Geometry check sheet. Reference: the model listing, model coordinates, mm. A direction names the side the tool comes from. Round coordinates to 2 decimals unless told otherwise and drop trailing zeros. Order: outer loops, then holes, each group sorted by start corner. A loop starts at its lowest first (then second) coordinate and runs counter-clockwise, first axis right, second up. Notation, with made-up numbers: (48, -30) - (63, -30) arc R19 cw to (63, -21) - close; hole circle Ø1 at (19, -34). An arc over 180 degrees is marked (long way). Use a Markdown table: item, result. Add a question column.
(1) Section check A-A on x = 18. Record the boundary of the cut face in (y, z).
(2) Section check C-C on z = 6.75. Record the boundary of the cut face in (x, y), then the cut area to 3 significant figures.
(3) Mould release check, pull along X, two halves, no side actions. Record for faces 1 (the face through (5, -49.229, 13)), 2 (the face through (-39.658, 38, 13)), 3 (the face through (-14, 120.636, 13)): released by +X, released by -X, zero draft, split by the parting line, or undercut.
(4) Access from +Z, -Z, +X, -X, +Y, -Y to the whole of each face (thin tool, end or side, straight path). Record for faces 4 (the face through (15, 40, 25.4)), 5 (the face through (-13, 103.174, 13)).
(5) Thickness scan on line 1 along Y through (x, z) = (-3, 10.75); line 2 along Y through (x, z) = (-16.5, 10.5); line 3 along Y through (x, z) = (3, 11.5). Record the ranges inside material, lowest first. Write a range as [from, to].
(6) Section check B-B on y = 0. Record the boundary of the cut face in (x, z).
```python
from build123d import *

# Parameters (mm, degrees)
F0_W     = 89.875921
F0_H     = 176.559519
F0_R     = 21.247903
F1_DEPTH = 25.4


with BuildPart() as f1:
    # F0 (on Top) → F1 (new body)
    with BuildSketch(Plane.XY):
        with Locations((5.27959, 39.050722)):
            Rectangle(F0_W, F0_H)
        with Locations((5.334, 19.290369)):
            Circle(F0_R, mode=Mode.SUBTRACT)
        with BuildLine():
            Line((-7.477125, 103.173869), (-19.383375, 103.173869))
            ThreePointArc((-19.383375, 103.173869), (-25.696058, 105.708611), (-28.502868, 111.905119))
            ThreePointArc((-28.502868, 111.905119), (-25.696058, 118.101627), (-19.383375, 120.636369))
            Line((-19.383375, 120.636369), (-7.477125, 120.636369))
            ThreePointArc((-7.477125, 120.636369), (-1.164442, 118.101627), (1.642368, 111.905119))
            ThreePointArc((1.642368, 111.905119), (-1.164442, 105.708611), (-7.477125, 103.173869))
        make_face(mode=Mode.SUBTRACT)
    extrude(amount=F1_DEPTH)


solid = f1.part
```
Check sheet entries:
| question | item | result |
|---|---|---|
| 1 | outline | (-49.23, 0) - (2.23, 0) - (2.23, 25.4) - (-49.23, 25.4) - close; (36.35, 0) - (127.33, 0) - (127.33, 25.4) - (36.35, 25.4) - close |
| 2 | outline | (-39.66, -49.23) - (50.22, -49.23) - (50.22, 127.33) - (-39.66, 127.33) - close; hole (-28.5, 111.91) arc R9.13 ccw to (-19.38, 103.17) - (-7.48, 103.17) arc R9.13 ccw to (1.64, 111.91) arc R9.13 ccw to (-7.48, 120.64) - (-19.38, 120.64) arc R9.13 ccw to start; hole circle Ø42.5 at (5.33, 19.29) |
| 2 | area | 14,000 mm2 |
| 3 | face 1 | zero draft |
| 3 | face 2 | released by -X |
| 3 | face 3 | undercut |
| 4 | face 4 | +Z, +X, -X, +Y, -Y |
| 4 | face 5 | +Z, -Z |
| 5 | line 1 | y = [-49.23, -0.25], [38.84, 104.35], [119.46, 127.33] |
| 5 | line 2 | y = [-49.23, 103.17], [120.64, 127.33] |
| 5 | line 3 | y = [-49.23, -1.83], [40.41, 127.33] |
| 6 | outline | (-39.66, 0) - (-3.57, 0) - (-3.57, 25.4) - (-39.66, 25.4) - close; (14.24, 0) - (50.22, 0) - (50.22, 25.4) - (14.24, 25.4) - close |
